from build123d import *

# Parameters (mm, degrees)
F0_W     = 134.533889
F0_H     = 130.701862
F1_DEPTH = 99.06
F2_T     = -5.08
F3_R     = 5.588
F4_DEPTH = 127
F5_W     = 127.2032
F5_H     = 13.716
F5_R     = 5.588
F6_DEPTH = 2.54


with BuildPart() as f1:
    # F0 (on Top) → F1 (new body)
    with BuildSketch(Plane.XY):
        with Locations((1.950313, -1.526598)):
            Rectangle(F0_W, F0_H)
    extrude(amount=F1_DEPTH)

    # F2
    f2_openings = [f1.faces().sort_by_distance(p)[0] for p in [
        (1.950312, -1.526598, 99.06),
    ]]
    offset(amount=F2_T, openings=f2_openings)

    # F3 (on face) → F4 (cut)
    with BuildSketch(Plane(origin=(0, 63.824333, 0), x_dir=(-1, 0, 0), z_dir=(0, 1, 0))):
        with Locations((-1.950312, 86.518437)):
            Circle(F3_R)
        with Locations((-21.000312, 86.518437)):
            Circle(F3_R)
        with Locations((-40.050312, 86.518437)):
            Circle(F3_R)
        with Locations((-59.100312, 86.518437)):
            Circle(F3_R)
        with Locations((17.099688, 86.518437)):
            Circle(F3_R)
        with Locations((36.149688, 86.518437)):
            Circle(F3_R)
        with Locations((55.199688, 86.518437)):
            Circle(F3_R)
    extrude(amount=-F4_DEPTH, mode=Mode.SUBTRACT)

    # F5 (on face) → F6 (cut)
    with BuildSketch(Plane(origin=(0, 63.824333, 0), x_dir=(-1, 0, 0), z_dir=(0, 1, 0))):
        with Locations((-1.950312, 86.518437)):
            Rectangle(F5_W, F5_H)
        with Locations((-1.950312, 86.518437)):
            Circle(F5_R, mode=Mode.SUBTRACT)
    extrude(amount=-F6_DEPTH, mode=Mode.SUBTRACT)


solid = f1.part
Input: part model. Units: mm. Frame: model coordinates. A direction names the side the tool comes from. Round coordinates to 2 decimals unless told otherwise and drop trailing zeros. Loops run counter-clockwise (first coordinate to the right, second up) from the corner with the lowest first, then second, coordinate; pieces in that order, holes last. Notation, with made-up numbers: (-4, 25.25) -> (18, 25.25) arc R16 cw to (18, 32.25) -> close; hole circle Ø3 at (38.5, 9). An arc over 180 degrees is marked (long way). Answer as a JSON object with one key per item and string values. Group by question number.
1) Draft query along Z for faces 1 (the flat face through (2.8, 61.284, 80.5)), 2 (the flat face through (-3, -64, 99.06)), 3 (the flat face through (1, 63.824, 38)). Return one class per face: +Z half, -Z half, draft (parallel to the pull), parting line (faces both ways), or undercut.
2) Section query A-A on x = 13. Output: boundary loops of the cut face in (y, z).
3) Section query C-C on y = 42. Output: boundary loops of the cut face in (x, z).
4) Section query D-D on x = -33.5. Output: boundary loops of the cut face in (y, z), plus the area to 3 significant figures.
5) Ray query, L1, parallel to X at y = -28, z = 42; L2, parallel to Y at x = -24, z = 77; L3, parallel to Y at x = -51.5, z = 81. Return the intervals inside material, ascending.
6) Pin query (flat end, axial travel): pin 1 (10 mm diameter, centred on x = 5, y = -22, fed in from +Z); pin 2 (1 mm diameter, centred on x = -28, y = 21.5, fed in from -Z); pin 3 (13 mm diameter, centred on x = -17.1, z = 86.52, fed in from +Y); pin 4 (10 mm diameter, centred on x = -55.2, z = 86.52, fed in from +Y). Return the tip coordinate at first contact, or that it passes through.
7) Reachability of faces 4 (the flat face through (1, 58.744, 51)), 5 (the flat face through (69.217, -2, 49)), 6 (the cylindrical face through (3.162, 60.032, 81.063)) from +Z, -Z, +X, -X, +Y, -Y: full face, straight path, thin tool, end or side. Return the list, or none.
8) Section query B-B on z = 33.5. Output: boundary loops of the cut face in (x, y), plus the area to 3 significant figures.
Reply:
{
 "1": {"face 1": "undercut", "face 2": "+Z half", "face 3": "draft"},
 "2": {"outline": "(-66.88, 0) -> (63.82, 0) -> (63.82, 79.66) -> (61.28, 79.66) -> (61.28, 93.38) -> (63.82, 93.38) -> (63.82, 99.06) -> (58.74, 99.06) -> (58.74, 5.08) -> (-61.8, 5.08) -> (-61.8, 99.06) -> (-66.88, 99.06) -> close"},
 "3": {"outline": "(-65.32, 0) -> (69.22, 0) -> (69.22, 99.06) -> (64.14, 99.06) -> (64.14, 88.94) arc R5.59 cw to (64.14, 84.1) -> (64.14, 5.08) -> (-60.24, 5.08) -> (-60.24, 84.1) arc R5.59 cw to (-60.24, 88.94) -> (-60.24, 99.06) -> (-65.32, 99.06) -> close"},
 "4": {"outline": "(-66.88, 0) -> (63.82, 0) -> (63.82, 79.66) -> (61.28, 79.66) -> (61.28, 81.6) -> (58.74, 81.6) -> (58.74, 5.08) -> (-61.8, 5.08) -> (-61.8, 81.6) -> (-63.18, 81.6) -> (-63.18, 91.44) -> (-61.8, 91.44) -> (-61.8, 99.06) -> (-66.88, 99.06) -> close; (58.74, 91.44) -> (61.28, 91.44) -> (61.28, 93.38) -> (63.82, 93.38) -> (63.82, 99.06) -> (58.74, 99.06) -> close", "area": "1,550 mm2"},
 "5": {"L1": "x = -65.32 to -60.24, 64.14 to 69.22", "L2": "y = -66.88 to -61.8, 58.74 to 63.82", "L3": "y = -66.88 to -61.8, 58.74 to 61.28"},
 "6": {"pin 1": "stops at z = 5.08", "pin 2": "stops at z = 0", "pin 3": "stops at y = 61.28", "pin 4": "stops at y = -63.18"},
 "7": {"face 4": "+Z", "face 5": "+Z, -Z, +X, +Y, -Y", "face 6": "+Y"},
 "8": {"outline": "(-65.32, -66.88) -> (69.22, -66.88) -> (69.22, 63.82) -> (-65.32, 63.82) -> close; hole (-60.24, -61.8) -> (64.14, -61.8) -> (64.14, 58.74) -> (-60.24, 58.74) -> close", "area": "2,590 mm2"}
}
